Input: dimensioned drawing with shaded views. Units: mm. Origin: part minimum x, y, z. A direction names the side the tool comes from. Give positions to 0.01 mm unless a question says otherwise; leave off trailing zeros. Order: outer loops, then holes, each group sorted by start corner. A loop starts at its lowest first (then second) coordinate and runs counter-clockwise, first axis right, second up. Notation, with made-up numbers: M 53,39 L 94,39 A27 cw 94,77 Z; hole C 41.5,87.25 d10. An arc over 180 degrees is marked long. Answer in a Markdown table with one row per item. Add a question column.
(1) Section query B-B, the plane y = 11. Return loops of the section in (x, z).
(2) Set-up query: the marked faces 1, 2 and 3. Return all of +Z, -Z, +X, -X, +Y, -Y with unobstructed straight access to the full face (end or side cutting, diameter ignored); none if empty.
(3) Material intervals for line 1 along Z through (x, y) = (4, 16.75); line 2 along Y through (x, z) = (33, 24); line 3 along X through (y, z) = (14.25, 44.5), sorted ascending.
(4) Pin query (flat end, axial travel): P1, Ø1, axis at y = 13.5, z = 45.5, coming from the -X side; P2, Ø6, axis at x = 16.5, z = 19, coming from the -Y side; P3, Ø4, axis at y = 13, z = 12.5, coming from the +X side. Return the tip coordinate at first contact, or that it passes through.
(5) Section query A-A, the plane x = 18. Return loops of the section in (y, z).
(6) Section query C-C, the plane y = 2.5. Return loops of the section in (x, z).
(7) Section query D-D, the plane z = 26.5. Return loops of the section in (x, y), plus the area to 3 significant figures.
(8) Mould query, pull axis Z, two halves, no side actions, for the marked faces 4, 5 and 6. Classes: pulls with the +Z half, pulls with the -Z half, needs draft (parallel to the pull), parting line crosses it, or undercut.
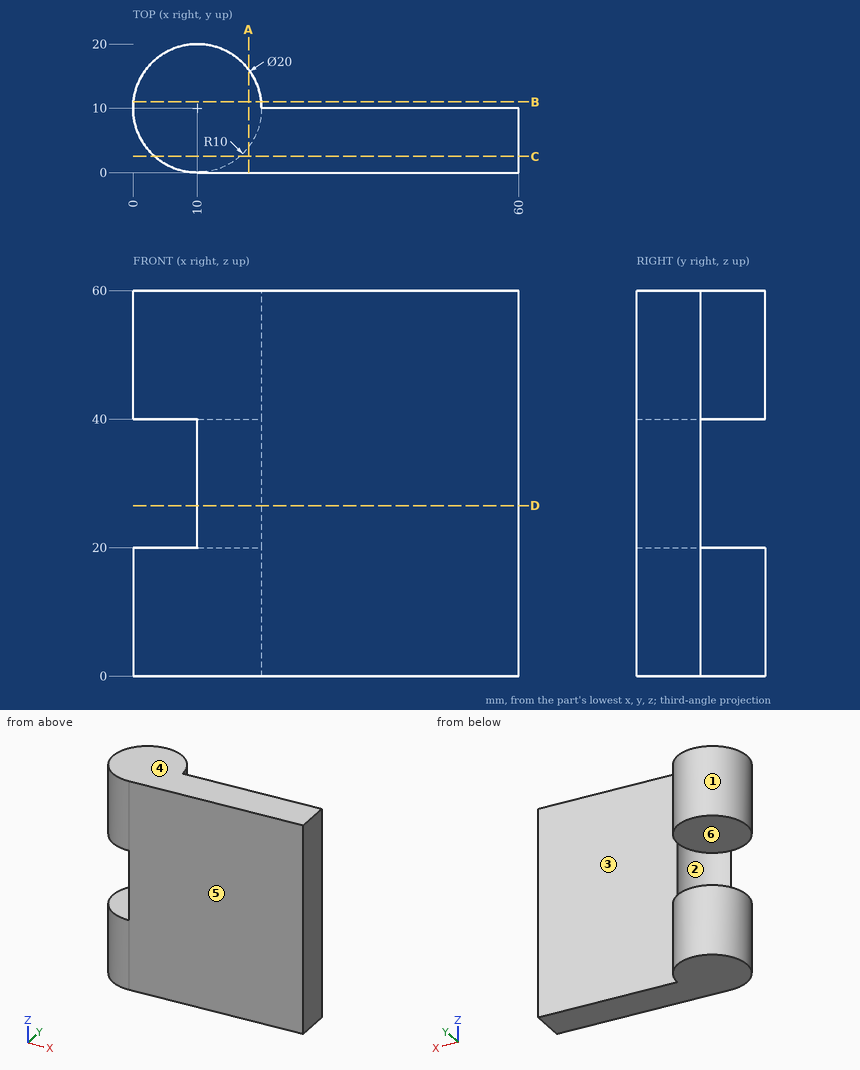
Values follow:
| question | item | result |
|---|---|---|
| 1 | outline | M 0.05,0 L 19.95,0 L 19.95,20 L 0.05,20 Z; M 0.05,40 L 19.95,40 L 19.95,60 L 0.05,60 Z |
| 2 | face 1 | +Z, -Z |
| 2 | face 2 | -X, +Y |
| 2 | face 3 | +Z, -Z, +X, +Y |
| 3 | line 1 | z = 0 to 20, 40 to 60 |
| 3 | line 2 | y = 0 to 10 |
| 3 | line 3 | x = 0.95 to 19.05 |
| 4 | P1 | stops at x = 0.46 |
| 4 | P2 | stops at y = 0 |
| 4 | P3 | stops at x = 19.95 |
| 5 | outline | M 0,0 L 16,0 L 16,20 L 4,20 L 4,40 L 16,40 L 16,60 L 0,60 Z |
| 6 | outline | M 3.39,0 L 60,0 L 60,60 L 3.39,60 L 3.39,40 L 16.61,40 L 16.61,20 L 3.39,20 Z |
| 7 | outline | M 10,0 L 60,0 L 60,10 L 20,10 A10 cw Z |
| 7 | area | 421 mm² |
| 8 | face 4 | pulls with the +Z half |
| 8 | face 5 | needs draft |
| 8 | face 6 | undercut |
